Could you check a few things on this drawing? It's one solid part, dimensions in mm from its lowest x, y, z. A direction names the side the tool comes from. Give positions to 0.01 mm unless a question says otherwise; leave off trailing zeros. Order: outer loops, then holes, each group sorted by start corner. A loop starts at its lowest first (then second) coordinate and runs counter-clockwise, first axis right, second up. Notation, with made-up numbers: M -25,61.25 L 2,61.25 A26 cw 2,92.25 Z; hole C 74,88 d8. An arc over 180 degrees is marked long. Use one line per item in the form item = value.
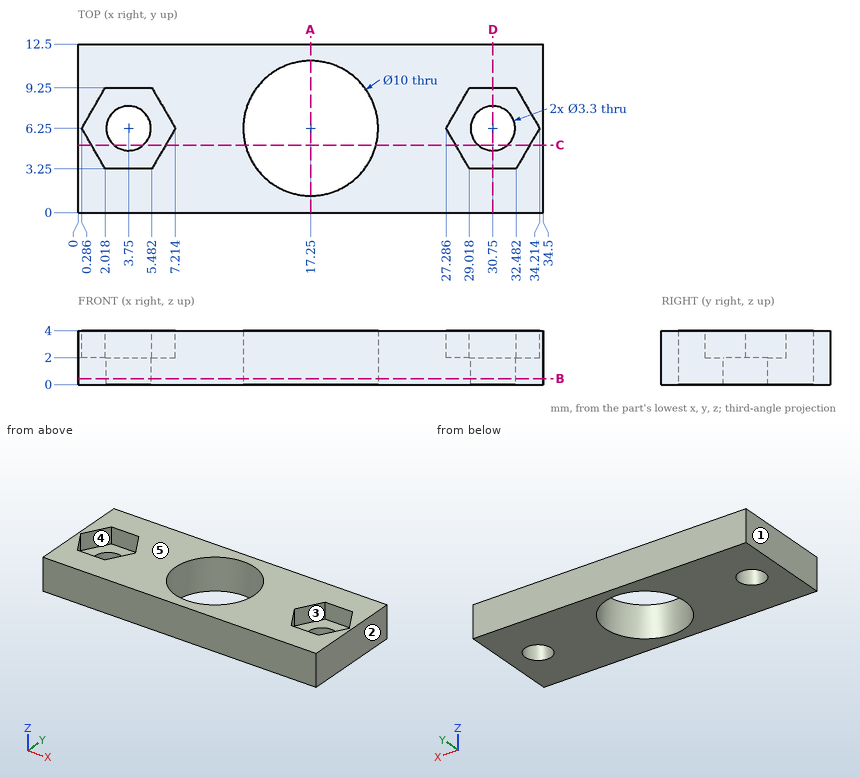
Q1. I'm going to push a flat-ended pin straight in: pin 1 Ø5.5 at (x, y) = (30.75, 6.25) entering from +Z. Where does the tip first touch, or does it pass through?
Found:
pin_1 = 2
Q2. On a 3-axis mill with a long thin cutter (end or side, diameter ignored), from which of +Z, -Z, +X, -X, +Y, -Y can I reach the whole of each face in a straight line? I mean the marked faces 4 and 5. Say none if no direction works.
Found:
face_4 = +Z
face_5 = +Z, +X, -X, +Y, -Y
Q3. I need wall thicknesses on L1, parallel to Y at x = 17.25, z = 1.5; L2, parallel to Y at x = 30.75, z = 1.4; L3, parallel to X at y = 5.5, z = 3.2. Which ranges of each line are inside material? Lowest first, please.
Found:
L1 = 0 to 1.25, 11.25 to 12.5
L2 = 0 to 4.6, 7.9 to 12.5
L3 = 0 to 0.72, 6.78 to 12.31, 22.19 to 27.72, 33.78 to 34.5
Q4. I want a section at A-A on x = 17.25. Write out the boundary of the cut face in (y, z).
Found:
outline = M 0,0 L 1.25,0 L 1.25,4 L 0,4 Z; M 11.25,0 L 12.5,0 L 12.5,4 L 11.25,4 Z
Q5. I want a section at D-D on x = 30.75. Write out the boundary of the cut face in (y, z), then the cut area to 3 significant figures.
Found:
outline = M 0,0 L 4.6,0 L 4.6,2 L 3.25,2 L 3.25,4 L 0,4 Z; M 7.9,0 L 12.5,0 L 12.5,4 L 9.25,4 L 9.25,2 L 7.9,2 Z
area = 31.4 mm²
Q6. I want a section at B-B on z = 0.45. Write out the boundary of the cut face in (x, y).
Found:
outline = M 0,0 L 34.5,0 L 34.5,12.5 L 0,12.5 Z; hole C 3.75,6.25 d3.3; hole C 17.25,6.25 d10; hole C 30.75,6.25 d3.3
Q7. I want a section at C-C on y = 5. Write out the boundary of the cut face in (x, z).
Found:
outline = M 0,0 L 2.67,0 L 2.67,2 L 1.01,2 L 1.01,4 L 0,4 Z; M 4.83,0 L 12.41,0 L 12.41,4 L 6.49,4 L 6.49,2 L 4.83,2 Z; M 22.09,0 L 29.67,0 L 29.67,2 L 28.01,2 L 28.01,4 L 22.09,4 Z; M 31.83,0 L 34.5,0 L 34.5,4 L 33.49,4 L 33.49,2 L 31.83,2 Z
Q8. Thinking about a two-plate mould opening in X: for the marked faces 1, 2 and 3, which applies, +X half, -X half, draft (parallel to the pull), parting line (faces both ways), or undercut?
Found:
face_1 = -X half
face_2 = +X half
face_3 = undercut
